Could you check a few things on this model? Use its own coordinates, in mm. A direction names the side the tool comes from. Give positions to 0.01 mm unless a question says otherwise; leave off trailing zeros. Write each loop counter-clockwise with the first axis right and the second up, starting at its lowest first coordinate (ties: lowest second). Pieces come first, ordered by that corner, then holes. Notation, with made-up numbers: M 84,47.25 L 110,47.25 A16 ccw 110,51.25 Z; hole C -16.75,-14.75 d8. An arc over 180 degrees is marked long. Answer as a JSON object with one key per item and string values. Group by question number.
```python
from build123d import *

# Parameters (mm, degrees)
SKETCH1_W           = 21.5
SKETCH1_H           = 21.5
SKETCH1_R           = 8
BOSS_EXTRUDE1_DEPTH = 2
SKETCH2_W           = 21.5
SKETCH2_H           = 21.5
SKETCH2_W_2         = 18.5
SKETCH2_H_2         = 18.5
BOSS_EXTRUDE2_DEPTH = 30
SKETCH3_W           = 27.5
SKETCH3_H           = 37.5
SKETCH3_R           = 1.5
SKETCH3_W_2         = 21.5
SKETCH3_H_2         = 21.5
BOSS_EXTRUDE3_DEPTH = 3
CUT_EXTRUDE1_DEPTH  = 3
CHAMFER1_SIZE       = 1
CHAMFER2_SIZE       = 2
SKETCH5_R           = 1.5
SKETCH5_R_2         = 1.45
BOSS_EXTRUDE4_DEPTH = 3
SKETCH6_R           = 10.75
SKETCH6_R_2         = 8
BOSS_EXTRUDE5_DEPTH = 1.5


with BuildPart() as part:
    # Sketch1 → Boss-Extrude1 (new body)
    with BuildSketch(Plane.XY):
        Rectangle(SKETCH1_W, SKETCH1_H)
        Circle(SKETCH1_R, mode=Mode.SUBTRACT)
    extrude(amount=BOSS_EXTRUDE1_DEPTH)

    # Sketch2 → Boss-Extrude2 (add)
    with BuildSketch(Plane.XY.offset(2)):
        Rectangle(SKETCH2_W, SKETCH2_H)
        Rectangle(SKETCH2_W_2, SKETCH2_H_2, mode=Mode.SUBTRACT)
    extrude(amount=BOSS_EXTRUDE2_DEPTH)

    # Sketch3 → Boss-Extrude3 (add)
    with BuildSketch(Plane.XY.offset(32)):
        Rectangle(SKETCH3_W, SKETCH3_H)
        with Locations((3.5, -15)):
            Circle(SKETCH3_R, mode=Mode.SUBTRACT)
        with Locations((3.5, 15)):
            Circle(SKETCH3_R, mode=Mode.SUBTRACT)
        with Locations((-8.5, 15)):
            Circle(SKETCH3_R, mode=Mode.SUBTRACT)
        with Locations((-8.5, -15)):
            Circle(SKETCH3_R, mode=Mode.SUBTRACT)
        Rectangle(SKETCH3_W_2, SKETCH3_H_2, mode=Mode.SUBTRACT)
    extrude(amount=-BOSS_EXTRUDE3_DEPTH)

    # Sketch4 → Cut-Extrude1 (cut)
    with BuildSketch(Plane.XZ.offset(10.75)):
        with BuildLine():
            Line((-1.5, 29), (-1.5, 27))
            ThreePointArc((-1.5, 27), (0, 25.5), (1.5, 27))
            Line((1.5, 27), (1.5, 29))
            Line((1.5, 29), (-1.5, 29))
        make_face()
    extrude(amount=-CUT_EXTRUDE1_DEPTH, mode=Mode.SUBTRACT)

    # Chamfer1
    chamfer1_edges = [part.edges().sort_by_distance(p)[0] for p in [
        (-10.75, 10.75, 14.5),
        (10.75, 10.75, 14.5),
        (10.75, -10.75, 14.5),
        (-10.75, -10.75, 14.5),
        (0, 10.75, 0),
        (10.75, 0, 0),
        (0, -10.75, 0),
        (-10.75, 0, 0),
    ]]
    chamfer(chamfer1_edges, length=CHAMFER1_SIZE)

    # Chamfer2
    chamfer2_edges = [part.edges().sort_by_distance(p)[0] for p in [
        (13.75, 18.75, 30.5),
        (13.75, -18.75, 30.5),
        (-13.75, -18.75, 30.5),
        (-13.75, 18.75, 30.5),
    ]]
    chamfer(chamfer2_edges, length=CHAMFER2_SIZE)

    # Sketch5 → Boss-Extrude4 (add)
    with BuildSketch(Plane(origin=(0, 0, 29), x_dir=(-1, 0, 0), z_dir=(0, 0, -1))):
        with Locations((8.5, -15)):
            Circle(SKETCH5_R)
        with Locations((8.5, -15)):
            Circle(SKETCH5_R_2, mode=Mode.SUBTRACT)
        with Locations((8.5, 15)):
            Circle(SKETCH5_R)
        with Locations((8.5, 15)):
            Circle(SKETCH5_R_2, mode=Mode.SUBTRACT)
    extrude(amount=-BOSS_EXTRUDE4_DEPTH)

    # Sketch6 → Boss-Extrude5 (add)
    with BuildSketch(Plane(origin=(0, 0, 0), x_dir=(-1, 0, 0), z_dir=(0, 0, -1))):
        Circle(SKETCH6_R)
        Circle(SKETCH6_R_2, mode=Mode.SUBTRACT)
    extrude(amount=-BOSS_EXTRUDE5_DEPTH)


solid = part.part
```
1) If we section it at D-D, the plane y = -6.5: List the corners of the cut face in (x, z) for me, plus the area to 3 significant figures.
2) If we section it at B-B, the plane z = 15: List the corners of the cut face in (x, y) for me.
3) Please list where these lines run through material, in increasing order: line 1 along Y through (x, z) = (3.5, 30.9); line 2 along Y through (x, z) = (-8.5, 31.1); line 3 along Y through (x, z) = (-1.25, 18). Write a range as from..to.
4) I'm going to push flat-ended pins straight in: pin 1 (15 mm diameter, centred on x = -4, z = 11, fed in from +Y); pin 2 (1.5 mm diameter, centred on y = 4.5, z = 24.5, fed in from +X); pin 3 (1.7 mm diameter, centred on x = -8.5, y = 15, fed in from +Z); pin 4 (9 mm diameter, centred on x = 0, z = 16, fed in from -Y). Where does each tip first touch, or does it pass through?
5) If we section it at A-A, the plane x = 3.5: List the corners of the cut face in (y, z) for me.
6) We'd pull the mould along Y, two halves only. Please class faces 1 (the flat face through (-8.4, 0.1, 2)), 2 (the flat face through (-10.75, 0, 15)), 3 (the flat face through (-10.3, 10.2, 15.2)): released by +Y, released by -Y, zero draft, split by the parting line, or undercut.
7) If we section it at C-C, the plane x = -8.5: List the corners of the cut face in (y, z) for me, plus the area to 3 significant figures.
8) For faces 4 (the flat face through (-6.03, 10.24, 0.49)), 5 (the flat face through (10.3, -10.2, 14.8)), 6 (the flat face through (10.75, 0, 15)), 7 (the flat face through (-1.5, -10, 28)), which set-ups out of +Z, -Z, +X, -X, +Y, -Y let a thin tool reach every point of the face, with its end or its side?
Taken from the geometry:
{
 "1": {"outline": "M -13.75,29 L -10.75,29 L -10.75,1 L -9.75,0 L -4.66,0 L -4.66,2 L -9.25,2 L -9.25,32 L -13.75,32 Z; M 4.66,0 L 9.75,0 L 10.75,1 L 10.75,29 L 13.75,29 L 13.75,32 L 9.25,32 L 9.25,2 L 4.66,2 Z", "area": "131 mm²"},
 "2": {"outline": "M -10.75,-9.75 L -9.75,-10.75 L 9.75,-10.75 L 10.75,-9.75 L 10.75,9.75 L 9.75,10.75 L -9.75,10.75 L -10.75,9.75 Z; hole M -9.25,-9.25 L 9.25,-9.25 L 9.25,9.25 L -9.25,9.25 Z"},
 "3": {"line 1": "-18.75..-16.5, -13.5..-9.25, 9.25..13.5, 16.5..18.75", "line 2": "-18.75..-16.45, -13.55..-9.25, 9.25..13.55, 16.45..18.75", "line 3": "-10.75..-9.25, 9.25..10.75"},
 "4": {"pin 1": "y = 10.75", "pin 2": "x = 10.75", "pin 3": "through", "pin 4": "y = -10.75"},
 "5": {"outline": "M -18.75,29 L -16.5,29 L -16.5,32 L -18.75,32 Z; M -13.5,29 L -10.75,29 L -10.75,1 L -10.16,0.41 L -10.16,0 L -7.19,0 L -7.19,2 L -9.25,2 L -9.25,32 L -13.5,32 Z; M 7.19,0 L 10.16,0 L 10.16,0.41 L 10.75,1 L 10.75,29 L 13.5,29 L 13.5,32 L 9.25,32 L 9.25,2 L 7.19,2 Z; M 16.5,29 L 18.75,29 L 18.75,32 L 16.5,32 Z"},
 "6": {"face 1": "undercut", "face 2": "zero draft", "face 3": "released by +Y"},
 "7": {"outline": "M -18.75,29 L -16.45,29 L -16.45,32 L -18.75,32 Z; M -13.55,29 L -10.75,29 L -10.75,1 L -9.75,0 L 9.75,0 L 10.75,1 L 10.75,29 L 13.55,29 L 13.55,32 L 9.25,32 L 9.25,2 L -9.25,2 L -9.25,32 L -13.55,32 Z; M 16.45,29 L 18.75,29 L 18.75,32 L 16.45,32 Z", "area": "163 mm²"},
 "8": {"face 4": "-Z, -X, +Y", "face 5": "-Z, +X, -Y", "face 6": "-Z, +X, +Y, -Y", "face 7": "-Y"}
}
